Geometry check sheet. Reference: the model listing, model coordinates, mm. Face numbers are marked on the shaded views. A direction names the side the tool comes from. Round coordinates to 2 decimals unless told otherwise and drop trailing zeros. Write each loop counter-clockwise with the first axis right and the second up, starting at its lowest first coordinate (ties: lowest second). Pieces come first, ordered by that corner, then holes.
Item 1: Scan lines: probe 1 along Y at (x, z) = (-0.5, 11.5); probe 2 along X at (y, z) = (-8.5, 8.5); probe 3 along Z at (x, y) = (4, -15). Record each from-to range of solid material in increasing order.
Item 2: Cross-section at D-D (z = 14). Enter the section's corners in (x, y), then the cut area to 3 significant figures.
Item 3: Access from +Z, -Z, +X, -X, +Y, -Y to the whole of each face (thin tool, end or side, straight path). Record for the marked faces 4 and 5.
Item 4: Draft check along X on the marked faces 1, 2 and 3. Enter one of: pulls with the +X half, pulls with the -X half, needs draft (parallel to the pull), parting line crosses it, or undercut.
Item 5: Cross-section at B-B (x = 0). Enter the section's corners in (y, z), then the cut area to 3 significant figures.
Item 6: Depth check by flat-ended pin: P1, Ø8, axis at x = -2.5, z = 9, coming from the -Y side; P2, Ø10, axis at x = 22.5, y = -5, coming from the +Z side; P3, Ø6, axis at x = 29, z = 10.5, coming from the +Y side; P4, Ø2, axis at x = -12.5, y = -8.5, coming from the -Z side. Enter the tip coordinate at first touch or a pass-through.
Item 7: Cross-section at A-A (z = 7.25). Enter the section's corners in (x, y).
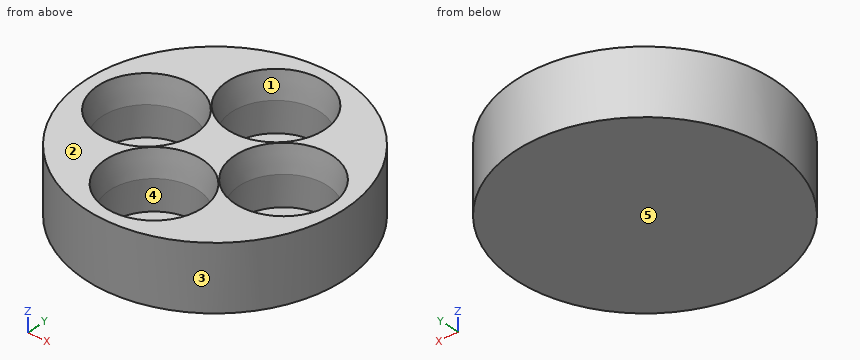
from build123d import *

# Parameters (mm, degrees)
F0_R       = 38.1
F0_R_2     = 3.175
F0_R_3     = 13
F1_DEPTH   = 19.05
F2_DEPTH   = 2.54
F3_SIZE2   = 1.27
F3_SIZE    = 7.62
F3_2_SIZE2 = 1.27
F3_2_SIZE  = 7.62
F3_3_SIZE2 = 1.27
F3_3_SIZE  = 7.62
F3_4_SIZE2 = 1.27
F3_4_SIZE  = 7.62


with BuildPart() as f1:
    # F0 (on Top) → F1 (new body)
    with BuildSketch(Plane.XY):
        Circle(F0_R)
        with Locations((-21.5526146906, -21.5526146906)):
            Circle(F0_R_2, mode=Mode.SUBTRACT)
        with Locations((0, -20.32)):
            Circle(F0_R_3, mode=Mode.SUBTRACT)
        with Locations((21.5526146906, -21.5526146906)):
            Circle(F0_R_2, mode=Mode.SUBTRACT)
        with Locations((-20.32, 0)):
            Circle(F0_R_3, mode=Mode.SUBTRACT)
        with Locations((-21.5526146906, 21.5526146906)):
            Circle(F0_R_2, mode=Mode.SUBTRACT)
        with Locations((20.32, 0)):
            Circle(F0_R_3, mode=Mode.SUBTRACT)
        with Locations((0, 20.32)):
            Circle(F0_R_3, mode=Mode.SUBTRACT)
        with Locations((21.5526146906, 21.5526146906)):
            Circle(F0_R_2, mode=Mode.SUBTRACT)
        with Locations((-21.5526146906, 21.5526146906)):
            Circle(F0_R_2)
        with Locations((-21.5526146906, -21.5526146906)):
            Circle(F0_R_2)
        with Locations((21.5526146906, -21.5526146906)):
            Circle(F0_R_2)
        with Locations((21.5526146906, 21.5526146906)):
            Circle(F0_R_2)
    extrude(amount=F1_DEPTH)

    # F0 (on Top) → F2 (join)
    with BuildSketch(Plane.XY):
        Circle(F0_R)
        with Locations((-21.5526146906, -21.5526146906)):
            Circle(F0_R_2, mode=Mode.SUBTRACT)
        with Locations((0, -20.32)):
            Circle(F0_R_3, mode=Mode.SUBTRACT)
        with Locations((21.5526146906, -21.5526146906)):
            Circle(F0_R_2, mode=Mode.SUBTRACT)
        with Locations((-20.32, 0)):
            Circle(F0_R_3, mode=Mode.SUBTRACT)
        with Locations((-21.5526146906, 21.5526146906)):
            Circle(F0_R_2, mode=Mode.SUBTRACT)
        with Locations((20.32, 0)):
            Circle(F0_R_3, mode=Mode.SUBTRACT)
        with Locations((0, 20.32)):
            Circle(F0_R_3, mode=Mode.SUBTRACT)
        with Locations((21.5526146906, 21.5526146906)):
            Circle(F0_R_2, mode=Mode.SUBTRACT)
        with Locations((-20.32, 0)):
            Circle(F0_R_3)
        with Locations((0, -20.32)):
            Circle(F0_R_3)
        with Locations((20.32, 0)):
            Circle(F0_R_3)
        with Locations((0, 20.32)):
            Circle(F0_R_3)
    extrude(amount=F2_DEPTH)

    # F3
    f3_edges = [f1.edges().sort_by_distance(p)[0] for p in [
        (-13, -20.32, 19.05),
    ]]
    f3_side = f1.faces().sort_by_distance((-13, -20.32, 10.795))[0]
    chamfer(f3_edges, length=F3_SIZE, length2=F3_SIZE2, reference=f3_side)

    # F3#2
    f3_2_edges = [f1.edges().sort_by_distance(p)[0] for p in [
        (-33.32, 0, 19.05),
    ]]
    f3_2_side = f1.faces().sort_by_distance((-33.32, 0, 10.795))[0]
    chamfer(f3_2_edges, length=F3_2_SIZE, length2=F3_2_SIZE2, reference=f3_2_side)

    # F3#3
    f3_3_edges = [f1.edges().sort_by_distance(p)[0] for p in [
        (-13, 20.32, 19.05),
    ]]
    f3_3_side = f1.faces().sort_by_distance((-13, 20.32, 10.795))[0]
    chamfer(f3_3_edges, length=F3_3_SIZE, length2=F3_3_SIZE2, reference=f3_3_side)

    # F3#4
    f3_4_edges = [f1.edges().sort_by_distance(p)[0] for p in [
        (7.32, 0, 19.05),
    ]]
    f3_4_side = f1.faces().sort_by_distance((7.32, 0, 10.795))[0]
    chamfer(f3_4_edges, length=F3_4_SIZE, length2=F3_4_SIZE2, reference=f3_4_side)


solid = f1.part
Resolved:
1. probe 1: y = -38.1 to -33.32, -7.32 to 7.32, 33.32 to 38.1
1. probe 2: x = -37.14 to -30.16, -10.48 to -5.41, 5.41 to 10.48, 30.16 to 37.14
1. probe 3: z = 0 to 2.54
2. outline: circle Ø76.2 at (0, 0); hole circle Ø26.86 at (-20.32, 0); hole circle Ø26.86 at (0, -20.32); hole circle Ø26.86 at (0, 20.32); hole circle Ø26.86 at (20.32, 0)
2. area: 2,290 mm2
3. face 4: +Z
3. face 5: -Z, +X, -X, +Y, -Y
4. face 1: undercut
4. face 2: needs draft
4. face 3: parting line crosses it
5. outline: (-38.1, 0) - (38.1, 0) - (38.1, 19.05) - (34.59, 19.05) - (33.32, 11.43) - (33.32, 2.54) - (7.32, 2.54) - (7.32, 11.43) - (6.05, 19.05) - (-6.05, 19.05) - (-7.32, 11.43) - (-7.32, 2.54) - (-33.32, 2.54) - (-33.32, 11.43) - (-34.59, 19.05) - (-38.1, 19.05) - close
5. area: 574 mm2
6. P1: stops at y = -38.1
6. P2: stops at z = 2.54
6. P3: stops at y = 27.85
6. P4: stops at z = 0
7. outline: circle Ø76.2 at (0, 0); hole circle Ø26 at (-20.32, 0); hole circle Ø26 at (0, -20.32); hole circle Ø26 at (0, 20.32); hole circle Ø26 at (20.32, 0)
